```python
from build123d import *

# Parameters (mm, degrees)
SKETCH1_W           = 100
SKETCH1_H           = 177.5
BOSS_EXTRUDE1_DEPTH = 2
SKETCH3_W           = 2
SKETCH3_H           = 20
BOSS_EXTRUDE2_DEPTH = 6
SKETCH4_W           = 96
SKETCH4_H           = 2
BOSS_EXTRUDE3_DEPTH = 4
BOSS_EXTRUDE5_DEPTH = 33
SKETCH7_W           = 18
SKETCH7_H           = 14
CUT_EXTRUDE2_DEPTH  = 207.386167172


with BuildPart() as part:
    # Sketch1 → Boss-Extrude1 (new body)
    with BuildSketch(Plane.XY):
        with Locations((50, 88.75)):
            Rectangle(SKETCH1_W, SKETCH1_H)
    extrude(amount=BOSS_EXTRUDE1_DEPTH)

    # Sketch3 → Boss-Extrude2 (add)
    with BuildSketch(Plane(origin=(0, 0, 0), x_dir=(-1, 0, 0), z_dir=(0, 0, -1))):
        Polygon((-98, 175.5), (-88, 175.5), (-88, 173.5), (-96, 173.5), (-96, 165.5), (-98, 165.5), align=None)
        Polygon((-12, 175.5), (-2, 175.5), (-2, 165.5), (-4, 165.5), (-4, 173.5), (-12, 173.5), align=None)
        Polygon((-2, 3), (-12, 3), (-12, 5), (-4, 5), (-4, 13), (-2, 13), align=None)
        with Locations((-97, 90.5)):
            Rectangle(SKETCH3_W, SKETCH3_H)
        with Locations((-3, 90.5)):
            Rectangle(SKETCH3_W, SKETCH3_H)
    extrude(amount=BOSS_EXTRUDE2_DEPTH)

    # Sketch4 → Boss-Extrude3 (add)
    with BuildSketch(Plane(origin=(0, 0, 0), x_dir=(-1, 0, 0), z_dir=(0, 0, -1))):
        with Locations((-50, 176.5)):
            Rectangle(SKETCH4_W, SKETCH4_H)
    extrude(amount=BOSS_EXTRUDE3_DEPTH)

    # Sketch5 → Boss-Extrude5 (add)
    with BuildSketch(Plane(origin=(0, 0, 0), x_dir=(-1, 0, 0), z_dir=(0, 0, -1))):
        Polygon((-98, 3), (-80, 3), (-80, 25), (-98, 25), (-98, 23), (-82, 23), (-82, 9), (-98, 9), align=None)
    extrude(amount=BOSS_EXTRUDE5_DEPTH)

    # Sketch7 → Cut-Extrude2 (cut, through all)
    with BuildSketch(Plane(origin=(0, 0, 0), x_dir=(-1, 0, 0), z_dir=(0, 0, -1))):
        with Locations((-91, 16)):
            Rectangle(SKETCH7_W, SKETCH7_H)
    extrude(amount=-CUT_EXTRUDE2_DEPTH, mode=Mode.SUBTRACT)


solid = part.part
```
Design review of the part built by this model. Coordinates are the model's own, in mm. A direction names the side the tool comes from. Coordinates: 2 decimals unless noted, no trailing zeros. Order: outer loops, then holes, each group sorted by start corner. A loop starts at its lowest first (then second) coordinate and runs counter-clockwise, first axis right, second up. Notation, with made-up numbers: (87.5, 26.5) - (120.5, 26.5) arc R31 ccw to (120.5, 59.5) - close; hole circle Ø11 at (68, 85). An arc over 180 degrees is marked (long way). Answer in a Markdown table with one row per item.
(1) For faces 4 (the flat face through (91, 23, -16)), 5 (the flat face through (4, 90, -3)), 6 (the flat face through (98, 171, -3)), 7 (the flat face through (7, 3, -3)), 8 (the flat face through (2, 8, -3)), list the 3-axis set-ups (+Z, -Z, +X, -X, +Y, -Y) from which the entire face can be reached by the end or side of a thin tool; tool diameter is ignored.
Checked values:
| item | result |
|---|---|
| face 4 | +Z, -Z, +X |
| face 5 | -Z |
| face 6 | -Z, +X, +Y, -Y |
| face 7 | -Z, +X, -X, -Y |
| face 8 | -Z, -X, +Y, -Y |
(2) Consider section D-D on x = 53. State the section outline as (y, z) points.
Checked values:
| item | result |
|---|---|
| outline | (0, 0) - (175.5, 0) - (175.5, -4) - (177.5, -4) - (177.5, 2) - (0, 2) - close |
(3) Wall thickness on line 1 along X through (y, z) = (97.5, -2); line 2 along Y through (x, z) = (95.5, -7.5); line 3 along Z through (x, y) = (50.5, 147.5): over which ranges is each line inside the solid? List them lowest first. Write a range as from..to.
Checked values:
| item | result |
|---|---|
| line 1 | 2..4, 96..98 |
| line 2 | 3..9, 23..25 |
| line 3 | 0..2 |
(4) Consider section B-B on y = 88.5. State the section outline as (x, z) points, plus the area to 3 significant figures.
Checked values:
| item | result |
|---|---|
| outline | (0, 0) - (2, 0) - (2, -6) - (4, -6) - (4, 0) - (96, 0) - (96, -6) - (98, -6) - (98, 0) - (100, 0) - (100, 2) - (0, 2) - close |
| area | 224 mm^2 |
(5) The part is to be moulded in two halves that separate along X. For faces 1 (the flat face through (92, 173.5, -3)), 2 (the flat face through (3.6, 5.8, -6)), 3 (the flat face through (98, 6, -16)), say which applies: released by +X, released by -X, zero draft, split by the parting line, or undercut.
Checked values:
| item | result |
|---|---|
| face 1 | undercut |
| face 2 | zero draft |
| face 3 | released by +X |
(6) Consider section A-A on x = 92. State the section outline as (y, z) points, plus the area to 3 significant figures.
Checked values:
| item | result |
|---|---|
| outline | (0, 0) - (3, 0) - (3, -33) - (9, -33) - (9, 2) - (0, 2) - close; (23, -33) - (25, -33) - (25, 0) - (173.5, 0) - (173.5, -6) - (175.5, -6) - (175.5, -4) - (177.5, -4) - (177.5, 2) - (23, 2) - close |
| area | 611 mm^2 |
(7) Clearance check with flat-ended pins moving along their axes: pin 1 (1.8 mm diameter, centred on x = 8.5, z = -2, fed in from -Y); pin 2 (2 mm diameter, centred on x = 53.5, z = -5.5, fed in from -Y); pin 3 (2 mm diameter, centred on y = 174.5, z = -3, fed in from +X); pin 4 (5 mm diameter, centred on x = 28, y = 153.5, fed in from -Z). State where each tip first meets the part, or that it passes through.
Checked values:
| item | result |
|---|---|
| pin 1 | y = 3 |
| pin 2 | through |
| pin 3 | x = 98 |
| pin 4 | z = 0 |
(8) Consider section C-C on z = -24. State the section outline as (x, y) points.
Checked values:
| item | result |
|---|---|
| outline | (80, 3) - (98, 3) - (98, 9) - (82, 9) - (82, 23) - (98, 23) - (98, 25) - (80, 25) - close |
